Build history of the part. All positions in model axes, mm. Give positions to 0.01 mm unless a question says otherwise; leave off trailing zeros. Write each loop counter-clockwise with the first axis right and the second up, starting at its lowest first coordinate (ties: lowest second). Pieces come first, ordered by that corner, then holes. Notation, with made-up numbers: (-6, 39) -> (15, 39) arc R14 ccw to (15, 52) -> close; hole circle Ø10 at (66.25, 20.25). An arc over 180 degrees is marked (long way). Write item = value, one per line. Start each with the question number.
Q1. Saw through at B-B, the plane y = -18.5. List the corners of the cut face in (x, z), then the cut area to 3 significant figures.
Q2. Saw through at A-A, the plane z = 1.15. List the corners of the cut face in (x, y).
Q3. Saw through at C-C, the plane x = 21. List the corners of the cut face in (y, z), then the cut area to 3 significant figures.
Q4. Wall check: line 1 (Y direction, x = 0.5, z = 0.1); line 2 (X direction, y = 0.5, z = 1.4); line 3 (X direction, y = -24, z = 0.7). Give the ranges that are in metal, low to high.
Q5. Drop a flat-ended pin along its axis: P1, Ø0.8, axis at y = -24, z = 0.5, coming from the +X side. Give the stop position or say it passes through.
from build123d import *

# Parameters (mm, degrees)
BOSS_EXTRUDE1_DEPTH = 1.6


with BuildPart() as part:
    # Sketch1 → Boss-Extrude1 (new body)
    with BuildSketch(Plane.XY):
        with BuildLine():
            Line((-23.5, -14.958275302), (-23.5, -30))
            ThreePointArc((-23.5, -30), (-22.035533906, -33.535533906), (-18.5, -35))
            Line((-18.5, -35), (18.5, -35))
            ThreePointArc((18.5, -35), (22.035533906, -33.535533906), (23.5, -30))
            Line((23.5, -30), (23.5, -14.958275302))
            ThreePointArc((23.5, -14.958275302), (23.773610701, -11.661372935), (24.586956522, -8.454677344))
            ThreePointArc((24.586956522, -8.454677344), (0, 26), (-24.586956522, -8.454677344))
            ThreePointArc((-24.586956522, -8.454677344), (-23.773610701, -11.661372935), (-23.5, -14.958275302))
        make_face()
    extrude(amount=BOSS_EXTRUDE1_DEPTH)


solid = part.part
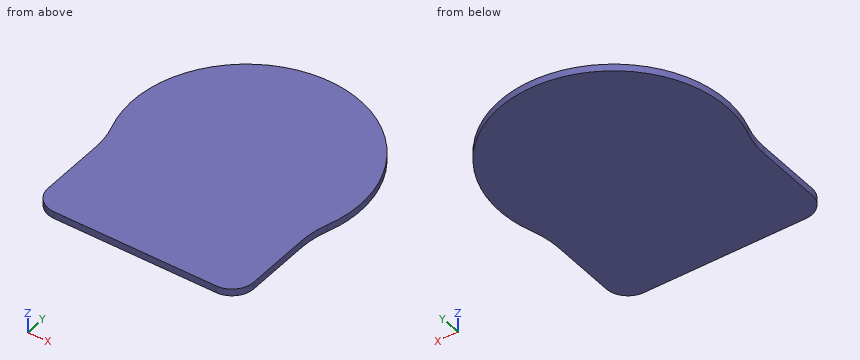
Report:
q1.outline = (-23.5, 0) -> (23.5, 0) -> (23.5, 1.6) -> (-23.5, 1.6) -> close
q1.area = 75.2 mm2
q2.outline = (-24.59, -8.45) arc R20 cw to (-23.5, -14.96) -> (-23.5, -30) arc R5 ccw to (-18.5, -35) -> (18.5, -35) arc R5 ccw to (23.5, -30) -> (23.5, -14.96) arc R20 cw to (24.59, -8.45) arc R26 ccw (long way) to start
q3.outline = (-34.33, 0) -> (15.33, 0) -> (15.33, 1.6) -> (-34.33, 1.6) -> close
q3.area = 79.5 mm2
q4.line_1 = -35 to 26
q4.line_2 = -26 to 26
q4.line_3 = -23.5 to 23.5
q5.P1 = 23.5
